Autodesk Inventor part; units mm, degrees
ref_plane "Start Plane" through (0, 0, 100) normal (0, 0, 1) x (1, 0, 0)
ref_plane "End Plane" through (0, 0, 1074.5) normal (0, 0, 1) x (1, 0, 0)
ref_plane "YZ Plane" through (0, 0, 0) normal (1, 0, 0) x (0, 1, 0)
ref_plane "Start Plane" through (0, 0, 100) normal (0, 0, 1) x (1, 0, 0)
ref_plane "End Plane" through (0, 0, 1074.5) normal (0, 0, 1) x (1, 0, 0)
sketch "Sketch" plane through (0, 0, 0) normal (0, 0, 1) x (1, 0, 0)
  line L0 (-25, -19) -> (-25, 19)
  line L1 (-19, 25) -> (19, 25)
  line L2 (25, 19) -> (25, -19)
  line L3 (19, -25) -> (-19, -25)
  arc A0 (-25, -19) -> (-19, -25) centre (-19, -19) ccw
  arc A1 (25, 19) -> (19, 25) centre (19, 19) ccw
  arc A2 (-19, 25) -> (-25, 19) centre (-19, 19) ccw
  arc A3 (19, -25) -> (25, -19) centre (19, -19) ccw
  arc A4 (-19, 22) -> (-22, 19) centre (-19, 19) ccw
  line L4 (-19, 22) -> (19, 22)
  arc A5 (22, 19) -> (19, 22) centre (19, 19) ccw
  line L5 (22, 19) -> (22, -19)
  arc A6 (19, -22) -> (22, -19) centre (19, -19) ccw
  line L6 (19, -22) -> (-19, -22)
  arc A7 (-22, -19) -> (-19, -22) centre (-19, -19) ccw
  line L7 (-22, -19) -> (-22, 19)
  line L8 (0, 36.7397) -> (0, -36.7397) construction
  line L9 (-36.7397, 0) -> (36.7397, 0) construction
  dimension "d7" = 6
  dimension "d9" = 50
  dimension "d11" = 50
  dimension "d12" = 3
  dimension "d15" = 25
  dimension "d16" = 25
extrude "Body" add sketch "Sketch" along normal up to surface (974.5 mm away) from surface at 100
sketch "Sketch3" plane through (0, 0, 0) normal (0, 0, 1) x (1, 0, 0)
  line L0 (0, 0) -> (10, 0)
ref_plane "Work Plane3" through (0, 0, 0) normal (0, -1, 0) x (1, 0, 0)
sketch "Sketch4" plane through (0, 0, 0) normal (0, -1, 0) x (1, 0, 0)
  line L0 (-2, 100) -> (12, 100)
  line L1 (-2, 1074.5) -> (12, 1074.5)
  dimension "d18" = 974.5
equation "\"d7\" = G_IR"
equation "\"d9\" = G_W"
equation "\"d11\" = G_H"
equation "\"d12\" = G_T"
equation "\"d15\" = 0.5 * d9"
equation "\"d16\" = 0.5 * d11"
equation "\"d3\" = G_L"
equation "\"G_W\" = 50"
equation "\"G_H\" = 50"
equation "\"G_T\" = 3"
equation "\"G_IR\" = 6"
equation "\"G_L\" = d18"
equation "\"G_OFFSET_END\" = 0"
equation "\"d14\" = G_OFFSET_END + B_L"
equation "\"B_L\" = 1074.5"
properties part number "ISO 4019 - 50x50x3 - 974.5" material "Steel, Mild"
Verification items for the finished model (mm, model axes). A direction names the side the tool comes from. Coordinates: 2 decimals unless noted, no trailing zeros. Write each loop counter-clockwise with the first axis right and the second up, starting at its lowest first coordinate (ties: lowest second). Pieces come first, ordered by that corner, then holes. Notation, with made-up numbers: M 13.25,-3.5 L 72.25,-3.5 A13 cw 72.25,5.5 Z; hole C 60.5,11 d4. An arc over 180 degrees is marked long. Answer as a JSON object with one key per item and string values. Group by question number.
(1) Material ranges on line 1 (Y direction, x = 14, z = 720); line 2 (X direction, y = 21, z = 672.5), recorded low to high.
(2) Release check for a two-part mould opening along Y. For faces 1 (the face through (0, 22, 580)), 2 (the face through (22, 0, 580)), 3 (the face through (0, 25, 580)), 4 (the face through (-22.3, 0.1, 100)) record: +Y half, -Y half, draft (parallel to the pull), parting line (faces both ways), or undercut.
(3) Cross-section at C-C, the plane z = 328. Record the cut outline in (x, y), and give its area (3 significant figures).
(4) Cross-section at A-A, the plane x = 0.5. Record the cut outline in (y, z).
(5) Tool access check on faces 5 (the face through (-22, 0, 580)), 6 (the face through (0, -25, 580)). Record the directions out of +Z, -Z, +X, -X, +Y, -Y that give a thin tool (end or side, any length) a straight path to the whole face; none if there is none.
Reply:
{
 "1": {"line 1": "-25 to -22, 22 to 25", "line 2": "-24.66 to -21.24, 21.24 to 24.66"},
 "2": {"face 1": "undercut", "face 2": "undercut", "face 3": "+Y half", "face 4": "draft"},
 "3": {"outline": "M -25,-19 A6 ccw -19,-25 L 19,-25 A6 ccw 25,-19 L 25,19 A6 ccw 19,25 L -19,25 A6 ccw -25,19 Z; hole M -22,-19 A3 ccw -19,-22 L 19,-22 A3 ccw 22,-19 L 22,19 A3 ccw 19,22 L -19,22 A3 ccw -22,19 Z", "area": "541 mm²"},
 "4": {"outline": "M -25,100 L -22,100 L -22,1074.5 L -25,1074.5 Z; M 22,100 L 25,100 L 25,1074.5 L 22,1074.5 Z"},
 "5": {"face 5": "+Z, -Z", "face 6": "+Z, -Z, +X, -X, -Y"}
}
